Source: CAD feature listing. Evaluate the final solid. Frame: model axes, mm. Coordinates: 2 decimals unless noted, no trailing zeros. Order: outer loops, then holes, each group sorted by start corner. A loop starts at its lowest first (then second) coordinate and runs counter-clockwise, first axis right, second up. Notation, with made-up numbers: (53.25, 55.25) -> (111.25, 55.25) arc R22 cw to (111.25, 74.25) -> close; hole circle Ø9 at (60.5, 38.5). An arc over 180 degrees is marked (long way). Write item = value, one per line. Start each with the question number.
Item 1: Section query A-A (z = 0.55). Output: boundary loops of the cut face in (x, y).
Item 2: Ray query, line 1 along X through (y, z) = (-7, -0.65); line 2 along Z through (x, y) = (-1.1, 6.25); line 3 along Z through (x, y) = (-1.8, -5.5). Return the intervals inside material, ascending. Write a range as [from, to].
Item 3: Section query C-C (y = -5.25). Output: boundary loops of the cut face in (x, z).
Item 4: Contact query for a flat-ended pin moving along its axis: pin 1 (3 mm diameter, centred on x = -1, y = 2, fed in from +Z). Output: stop coordinate, or through.
Item 5: Section query B-B (x = 1.4). Output: boundary loops of the cut face in (y, z), then the cut area to 3 significant figures.
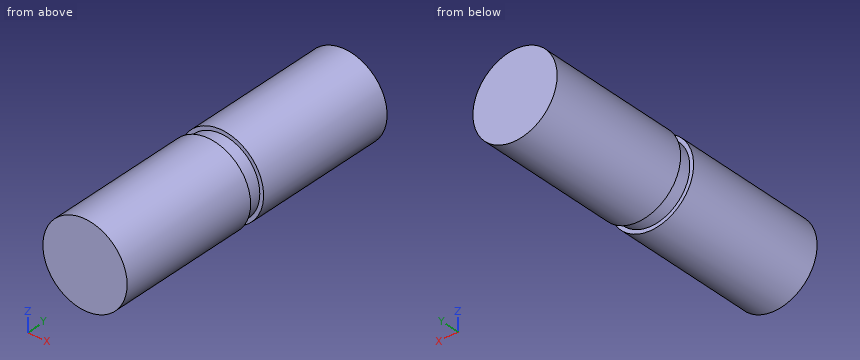
```python
from build123d import *

# Parameters (mm, degrees)
F0_R     = 2.5
F1_DEPTH = 1
F2_R     = 2.75
F3_DEPTH = 9.5
F4_R     = 2.75
F5_DEPTH = 9.5


with BuildPart() as f1:
    # F0 (on Front) → F1 (new body)
    with BuildSketch(Plane.XZ):
        Circle(F0_R)
    extrude(amount=F1_DEPTH)

    # F2 (on face) → F3 (join)
    with BuildSketch(Plane(origin=(0, 0, 0), x_dir=(-1, 0, 0), z_dir=(0, 1, 0))):
        Circle(F2_R)
    extrude(amount=F3_DEPTH)

    # F4 (on face) → F5 (join)
    with BuildSketch(Plane.XZ.offset(1)):
        Circle(F4_R)
    extrude(amount=F5_DEPTH)


solid = f1.part
```
Computed:
q1.outline = (-2.69, -10.5) -> (2.69, -10.5) -> (2.69, -1) -> (2.44, -1) -> (2.44, 0) -> (2.69, 0) -> (2.69, 9.5) -> (-2.69, 9.5) -> (-2.69, 0) -> (-2.44, 0) -> (-2.44, -1) -> (-2.69, -1) -> close
q2.line_1 = [-2.67, 2.67]
q2.line_2 = [-2.52, 2.52]
q2.line_3 = [-2.08, 2.08]
q3.outline = circle Ø5.5 at (0, 0)
q4.pin_1 = 2.75
q5.outline = (-10.5, -2.37) -> (-1, -2.37) -> (-1, -2.07) -> (0, -2.07) -> (0, -2.37) -> (9.5, -2.37) -> (9.5, 2.37) -> (0, 2.37) -> (0, 2.07) -> (-1, 2.07) -> (-1, 2.37) -> (-10.5, 2.37) -> close
q5.area = 94.1 mm^2
